Study the drawing (mm; zero at the part's minimum x, y, z) and answer. A direction names the side the tool comes from. Give positions to 0.01 mm unless a question says otherwise; leave off trailing zeros. Order: outer loops, then holes, each group sorted by start corner. A loop starts at its lowest first (then second) coordinate and runs counter-clockwise, first axis right, second up.
Item 1: A cutting plane is placed at A-A (z = 7). State how many separate pieces and enclosed holes the cut face has, plus the area to 3 significant figures.
Item 2: A cutting plane is placed at D-D (y = 4.5). Write down the section's boundary in (x, z).
Item 3: The mould has two halves that part along Y. Classify the marked faces 5, 6 and 7: +Y half, -Y half, draft (parallel to the pull), parting line (faces both ways), or undercut.
Item 4: Which of the six approach directions +Z, -Z, +X, -X, +Y, -Y give full straight-line access (tool end or side, diameter ignored) to the marked faces 1, 2, 3 and 4?
Item 5: Find the intervals of material crossed by line 1 along X through (y, z) = (4.05, 7); line 2 along Z through (x, y) = (4.5, 7); line 3 along X through (y, z) = (1.75, 6.75), in increasing order.
Item 6: A cutting plane is placed at B-B (y = 12.75). Write down the section's boundary in (x, z), plus the area to 3 significant figures.
Item 7: Given pin 1 Ø1.5 at (x, z) = (1.5, 5) entering from +Y; pin 2 Ø3 at (x, z) = (6.5, 7) entering from +Y; pin 3 Ø4 at (y, z) = (3.5, 9) entering from +X; pin 4 Ø1.8 at (y, z) = (7, 7) entering from +X, each flat-ended and moving along its own axis, determine where each tip first touches the part or whether it passes through.
Item 8: A cutting plane is placed at C-C (x = 12.25). Write down the section's boundary in (y, z).
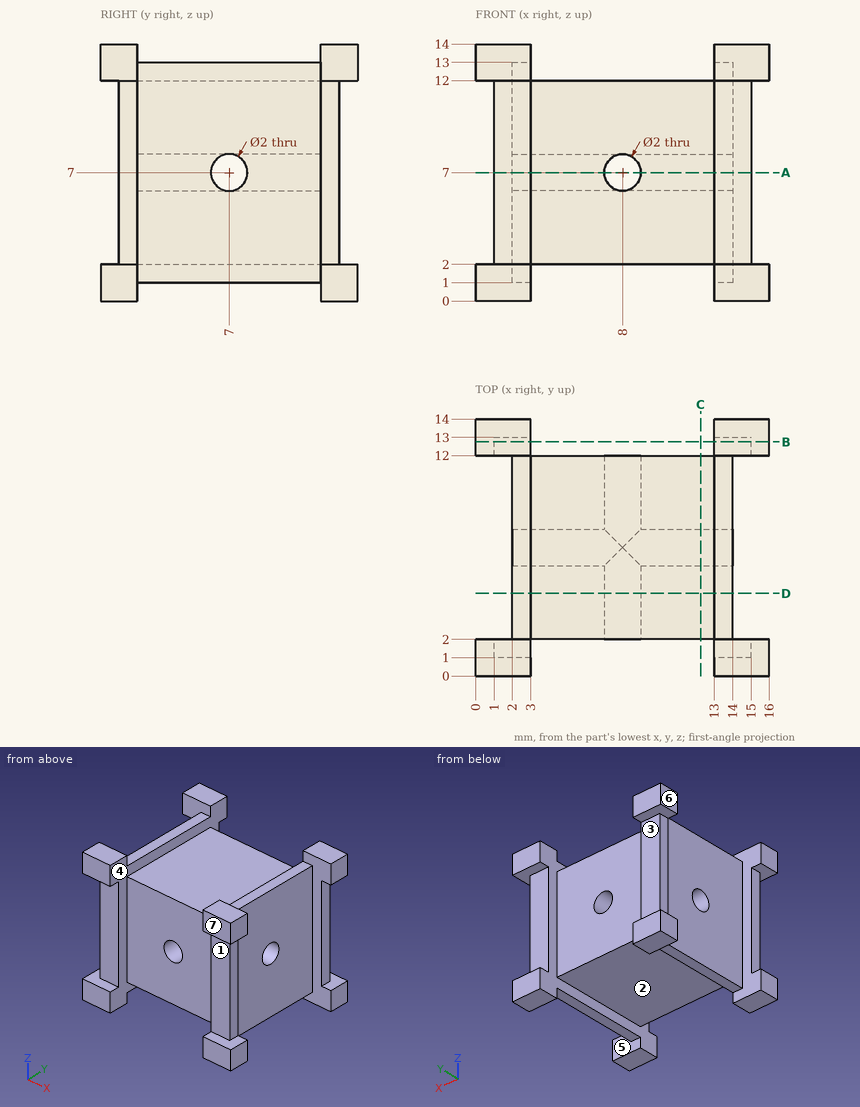
Response values:
1. separate pieces: 4
1. enclosed holes: 0
1. area: 88.0 mm2
2. outline: (2, 1) - (3, 1) - (3, 2) - (13, 2) - (13, 1) - (14, 1) - (14, 13) - (13, 13) - (13, 12) - (3, 12) - (3, 13) - (2, 13) - close; hole circle Ø2 at (8, 7)
3. face 5: undercut
3. face 6: draft
3. face 7: -Y half
4. face 1: +X, -X, -Y
4. face 2: -Z, +Y, -Y
4. face 3: +X, -X, +Y
4. face 4: none
5. line 1: x = 2 to 7, 9 to 14
5. line 2: z = 2 to 6, 8 to 12
5. line 3: x = 1 to 3, 13 to 15
6. outline: (0, 0) - (3, 0) - (3, 14) - (0, 14) - (0, 12) - (1, 12) - (1, 2) - (0, 2) - close; (13, 0) - (16, 0) - (16, 2) - (15, 2) - (15, 12) - (16, 12) - (16, 14) - (13, 14) - close
6. area: 64.0 mm2
7. pin 1: stops at y = 13
7. pin 2: stops at y = 12
7. pin 3: stops at x = 15
7. pin 4: passes through
8. outline: (2, 2) - (12, 2) - (12, 12) - (2, 12) - close; hole circle Ø2 at (7, 7)
